Input: part model. Units: mm. Frame: model coordinates. Face numbers are marked on the shaded views. A direction names the side the tool comes from. Round coordinates to 2 decimals unless told otherwise and drop trailing zeros. Loops run counter-clockwise (first coordinate to the right, second up) from the corner with the lowest first, then second, coordinate; pieces in that order, holes last.
1) Access query for the marked faces 1, 2, 3 and 4. Directions: +Z, -Z, +X, -X, +Y, -Y. A direction counts if a zero-diameter tool reaches every point of the face in a straight line with its end or side. Return the directions, or none.
2) Ray query, line 1 along Y through (x, z) = (0, -1.75) (3 decimals); line 2 along X through (y, z) = (-8.5, -7.25); line 3 along X through (y, z) = (-9, -6). Return the intervals inside material, ascending.
3) Draft query along Y for the marked faces 5, 6 and 7. Return one class per face: pulls with the +Y half, pulls with the -Y half, needs draft (parallel to the pull), parting line crosses it, or undercut.
4) First-contact query: pin 1 (4.5 mm diameter, centred on x = 22, y = 1.5, fed in from +Z); pin 2 (5 mm diameter, centred on x = 23, z = -4.5, fed in from +Y); pin 3 (4 mm diameter, centred on x = 6, z = -3, fed in from -Y); pin 4 (1.5 mm diameter, centred on x = -6, z = -1, fed in from -Y). Flat tips, straight axial feed; report the tip coordinate or a pass-through.
5) Section A-A, the plane z = -3. Return loops of the section in (x, y) (3 decimals).
6) Section C-C, the plane y = -18.5. Return loops of the section in (x, z), and give its area (3 significant figures).
7) Section D-D, the plane x = -20.5. Return loops of the section in (y, z).
from build123d import *

# Parameters (mm, degrees)
SKETCH009_R     = 70.710678
POCKET004_DEPTH = 9
SKETCH010_R     = 4.5
POCKET005_DEPTH = 3
CHAMFER003_SIZE = 2
SKETCH013_W     = 3
SKETCH013_H     = 9
GROOVE002_ANGLE = 281.954395


with BuildPart() as part:
    # Sketch008 → Revolution002 (revolve)
    with BuildSketch(Plane.XZ):
        Polygon((70.710678, 0), (26.95, 0), (26, 0.95), (25.05, 0), (25, 0), (25, -7.5), (14, -7.5), (13.740136, -5.5), (12.116995, -5.5), (12.116995, -4.5), (5, -4.5), (5, 0), (3.975, 0), (2.025, 1.95), (2.025, -9), (70.710678, -9), align=None)
    revolve(axis=Axis((0, 0, 0), (0, 0, 1)))

    # Sketch012 → Revolution004 (revolve)
    with BuildSketch(Plane.XZ):
        Polygon((31.6, 1.95), (33.6, 1.95), (35.55, 0), (31.6, 0), align=None)
    revolve(axis=Axis((31.6, 0, 13.931554), (0, 0, -1)))

    # Sketch011 → Revolution003 (revolve)
    with BuildSketch(Plane.XZ):
        Polygon((42, 0), (42, 1.95), (44, 1.95), (45.95, 0), align=None)
    revolve(axis=Axis((42, 0, 13.737844), (0, 0, -1)))

    # Sketch009 → Pocket004 (cut, symmetric)
    with BuildSketch(Plane.XY):
        Circle(SKETCH009_R)
        with BuildLine():
            Line((20.976177, 17), (27, 17))
            Line((27, 17), (27, -17))
            Line((27, -17), (20.976177, -17))
            ThreePointArc((20.976177, 17), (-27, 0), (20.976177, -17))
        make_face(mode=Mode.SUBTRACT)
    extrude(amount=POCKET004_DEPTH, both=True, mode=Mode.SUBTRACT)

    # Sketch010 → Pocket005 (cut)
    with BuildSketch(Plane.XY.offset(-9)):
        Circle(SKETCH010_R)
    extrude(amount=POCKET005_DEPTH, mode=Mode.SUBTRACT)

    # Chamfer003
    chamfer003_edges = [part.edges().sort_by_distance(p)[0] for p in [
        (-2.025, 0, -6),
    ]]
    chamfer(chamfer003_edges, length=CHAMFER003_SIZE)

    # Sketch013 → Groove002 (revolve, symmetric, cut)
    with BuildSketch(Plane.XZ) as groove002_sk:
        with Locations((-25.5, 0)):
            Rectangle(SKETCH013_W, SKETCH013_H)
    revolve(axis=Axis((0, 0, 0), (0, 0, 1)), revolution_arc=GROOVE002_ANGLE / 2, mode=Mode.SUBTRACT)
    revolve(groove002_sk.sketch, axis=Axis((0, 0, 0), (0, 0, -1)), revolution_arc=GROOVE002_ANGLE / 2, mode=Mode.SUBTRACT)

    # Sketch017 → Groove004 (revolve, cut)
    with BuildSketch(Plane.XZ):
        Polygon((42, -7), (44, -7), (46, -9), (42, -9), align=None)
    revolve(axis=Axis((42, 0, 18.984909), (0, 0, -1)), mode=Mode.SUBTRACT)

    # Sketch018 → Groove005 (revolve, cut)
    with BuildSketch(Plane.XZ):
        Polygon((31.6, -7), (33.6, -7), (35.6, -9), (31.6, -9), align=None)
    revolve(axis=Axis((31.6, 0, 19.891285), (0, 0, -1)), mode=Mode.SUBTRACT)


solid = part.part
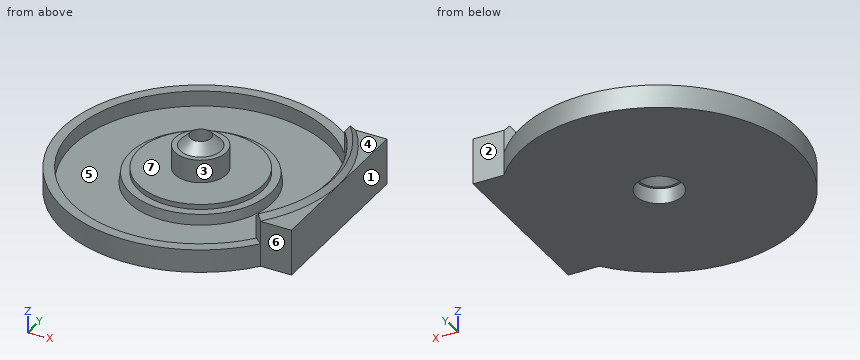
Final values:
1. face 1: +Z, -Z, +X, +Y, -Y
1. face 2: +Z, -Z, +X, +Y
1. face 3: +Z
1. face 4: +Z, +X
2. line 1: y = -5 to -2.025, 2.025 to 5
2. line 2: x = -25.63 to -23.51, -11.08 to 11.08, 23.51 to 27
2. line 3: x = -25.46 to -23.32, -10.47 to 10.47, 23.32 to 27
3. face 5: undercut
3. face 6: pulls with the -Y half
3. face 7: needs draft
4. pin 1: stops at z = -7.5
4. pin 2: stops at y = 17.57
4. pin 3: stops at y = -26.59
4. pin 4: passes through
5. outline: circle Ø10 at (0, 0); (19.422, -15.741) - (20.976, -17) - (27, -17) - (27, 17) - (20.976, 17) - (19.422, 15.741) arc R25 cw to start; hole circle Ø4.05 at (0, 0)
6. outline: (-19.67, -9) - (19.67, -9) - (19.67, -4.5) - (16.82, -4.5) - (16.82, -7.5) - (-16.82, -7.5) - (-16.82, -4.5) - (-19.67, -4.5) - close
6. area: 76.1 mm2
7. outline: (-17.57, -9) - (17.57, -9) - (17.57, -4.5) - (14.31, -4.5) - (14.31, -7.5) - (-14.31, -7.5) - (-14.31, -4.5) - (-17.57, -4.5) - close
